Here's how the part is built. I have some questions about the finished solid (model axes, mm). Face numbers are marked on the shaded views. A direction names the side the tool comes from. Round coordinates to 2 decimals unless told otherwise and drop trailing zeros. Write each loop counter-clockwise with the first axis right and the second up, starting at its lowest first coordinate (ties: lowest second). Pieces come first, ordered by that corner, then holes. Notation, with made-up numbers: (37.5, -18) -> (60.5, -18) arc R26 ccw to (60.5, 15) -> close; hole circle Ø2 at (46.5, 3). An arc over 180 degrees is marked (long way). Answer in a Markdown table with one row per item. Add a question column.
from build123d import *

# Parameters (mm, degrees)
F1_DEPTH    = 152.4
F2_T        = 2.54
F2_T3_DEPTH = 157.48


# Not quite as in the source:
# - a shell that OpenCascade refuses in one call is made with other operations: the cavity is built on its own and cut out


with BuildPart() as f1:
    # F0 (on Front) → F1 (new body)
    with BuildSketch(Plane.XZ):
        with BuildLine():
            Line((-37.8300789744, -10.7009902054), (-48.2259040094, -10.7009902054))
            Line((-48.2259040094, -10.7009902054), (-48.2259040094, -7.2357404328))
            ThreePointArc((-48.2259040094, -7.2357404328), (-49.0552526275, -5.8106548767), (-50.7040085729, -5.8277371868))
            Line((-50.7040085729, -5.8277371868), (-59.5905011949, -11.123357617))
            ThreePointArc((-59.5905011949, -11.123357617), (-61.8609001823, -13.4412951055), (-62.6898407936, -16.578236805))
            Line((-62.6898407936, -16.578236805), (-62.6898407936, -27.3817684501))
            Line((-62.6898407936, -27.3817684501), (-43.5946621001, -27.3817684501))
            Line((-43.5946621001, -27.3817684501), (-43.5946621001, -19.9903684501))
            Line((-43.5946621001, -19.9903684501), (0, -19.9903684501))
            Line((0, -19.9903684501), (0, -27.3817684501))
            Line((0, -27.3817684501), (16.9334635139, -27.3817684501))
            Line((16.9334635139, -27.3817684501), (16.9334635139, 48.305941894))
            ThreePointArc((16.9334635139, 48.305941894), (15.0735915744, 52.7960699546), (10.5834635139, 54.655941894))
            Line((10.5834635139, 54.655941894), (6.1501904505, 54.655941894))
            ThreePointArc((6.1501904505, 54.655941894), (2.3177679163, 53.3690474153), (0.0387070827, 50.0299694591))
            Line((0.0387070827, 50.0299694591), (-17.0932790838, -10.7009902054))
            Line((-17.0932790838, -10.7009902054), (-28.2165445387, -10.7009902054))
            Line((-28.2165445387, -10.7009902054), (-28.2165445387, -14.6972788498))
            Line((-28.2165445387, -14.6972788498), (-37.8300789744, -14.6972788498))
            Line((-37.8300789744, -14.6972788498), (-37.8300789744, -10.7009902054))
        make_face()
    extrude(amount=F1_DEPTH)

    # F2: shell of thickness 2.54, made by hand


with BuildPart() as f2_core1:
    # F2_t2: copy of F1
    add(f1.part)

    # the walls: a layer under each face that stays
    f2_faces = [f2_core1.faces().sort_by_distance(p)[0] for p in [
        (-8.5272860005, -76.2, 19.6644896269),
        (-22.6549118113, -76.2, -10.7009902054),
        (-28.2165445387, -76.2, -12.6991345276),
        (-33.0233117566, -76.2, -14.6972788498),
        (-37.8300789744, -76.2, -12.6991345276),
        (-43.0279914919, -76.2, -10.7009902054),
        (-48.2259040094, -76.2, -8.9683653191),
        (-55.1472548839, -76.2, -8.4755474019),
        (-61.8609001823, -76.2, -13.4412951055),
        (-62.6898407936, -76.2, -21.9800026276),
        (-53.1422514468, -76.2, -27.3817684501),
        (-43.5946621001, -76.2, -23.6860684501),
        (-21.79733105, -76.2, -19.9903684501),
        (0, -76.2, -23.6860684501),
        (8.4667317569, -76.2, -27.3817684501),
        (16.9334635139, -76.2, 10.4620867219),
        (15.0735915744, -76.2, 52.7960699546),
        (8.3668269822, -76.2, 54.655941894),
        (2.3177679163, -76.2, 53.3690474153),
    ]]
    thicken(f2_faces, amount=-F2_T, mode=Mode.SUBTRACT)

    # F2_s4 → F2_t3 (cut)
    with BuildSketch(Plane.XZ.offset(-2.54)):
        Polygon((-17.1177250172, -10.6686940951), (-14.6486857366, -11.3906012314), (-15.1706738376, -13.2409902054), (-17.0932790838, -13.2409902054), align=None)
        Polygon((-28.2419445387, -14.6718788498), (-25.6765445387, -14.6972788498), (-25.6765445387, -17.2372788498), (-28.2165445387, -17.2372788498), align=None)
        Polygon((-37.8046789744, -14.6718788498), (-37.8300789744, -17.2372788498), (-40.3700789744, -17.2372788498), (-40.3700789744, -14.6972788498), align=None)
        Polygon((-48.2005040094, -10.6755902054), (-48.2259040094, -13.2409902054), (-50.7659040094, -13.2409902054), (-50.7659040094, -10.7009902054), align=None)
        Polygon((-43.5692621001, -20.0157684501), (-46.1346621001, -19.9903684501), (-46.1346621001, -17.4503684501), (-43.5946621001, -17.4503684501), align=None)
        Polygon((-0.0254, -20.0157684501), (0, -17.4503684501), (2.54, -17.4503684501), (2.54, -19.9903684501), align=None)
    extrude(amount=F2_T3_DEPTH, mode=Mode.SUBTRACT)


with BuildPart() as f1_1:
    add(f1.part)

    # what is left inside the walls is the cavity
    f2_cavity = [f2_core1.part.solids().sort_by_distance(p)[0] for p in [
        (14.368064, -101.6, 11.732087),
    ]]
    add(f2_cavity, mode=Mode.SUBTRACT)


solid = f1_1.part
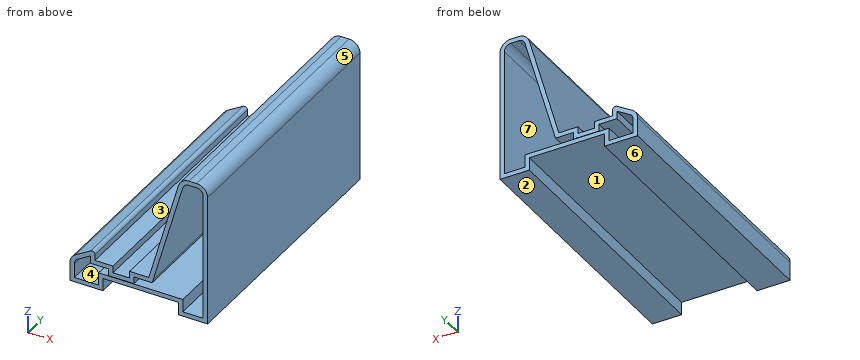
Item 1: On a 3-axis mill with a long thin cutter (end or side, diameter ignored), from which of +Z, -Z, +X, -X, +Y, -Y can I reach the whole of each face in a straight line? I mean the marked faces 1, 2, 3 and 4. Say none if no direction works.
Item 2: I need wall thicknesses on line 1 along X through (y, z) = (-89.5, -23); line 2 along Z through (x, y) = (-22.5, -11); line 3 along X through (y, z) = (-123, -9). Which ranges of each line are inside material? Lowest first, please. Write a range as from..to.
Item 3: If we section it at A-A on x = -2: Please give me the cut outline in (y, z), then the cut area to 3 significant figures.
Item 4: If we mould it in two halves opening along Z, with no side actions, what happens to the marked faces 5, 6 and 7? For each: pulls with the +Z half, pulls with the -Z half, needs draft (parallel to the pull), parting line crosses it, or undercut.
Item 5: For P1, Ø10, axis at x = -15, y = -64.5, coming from the -Z side; P2, Ø3.5, axis at y = -110.5, z = -12, coming from the -X side; P3, Ø11, axis at x = -56, y = -98, coming from the +Z side, each with a flat end and sliding along its axis, tell me the tip position at first contact or that it passes through.
Item 6: If we section it at B-B on z = 2.5: Please give me the cut outline in (x, y).
Results list:
| question | item | result |
|---|---|---|
| 1 | face 1 | -Z, +Y, -Y |
| 1 | face 2 | -Z, +X, -X, +Y, -Y |
| 1 | face 3 | +Z, +Y, -Y |
| 1 | face 4 | +Y, -Y |
| 2 | line 1 | -62.69..-60.15, -46.13..-43.59, 0..2.54, 14.39..16.93 |
| 2 | line 2 | -19.99..-17.45, -13.24..-10.7 |
| 2 | line 3 | -56.03..-51.07, -50.77..-48.23, -16.61..-13.97, 14.39..16.93 |
| 3 | outline | (-152.4, -19.99) -> (0, -19.99) -> (0, -17.45) -> (-152.4, -17.45) -> close; (-152.4, 33.45) -> (0, 33.45) -> (0, 42.8) -> (-152.4, 42.8) -> close |
| 3 | area | 1,810 mm² |
| 4 | face 5 | pulls with the +Z half |
| 4 | face 6 | pulls with the -Z half |
| 4 | face 7 | undercut |
| 5 | P1 | z = -19.99 |
| 5 | P2 | x = -62.03 |
| 5 | P3 | z = -5.72 |
| 6 | outline | (-13.37, -152.4) -> (-10.73, -152.4) -> (-10.73, 0) -> (-13.37, 0) -> close; (14.39, -152.4) -> (16.93, -152.4) -> (16.93, 0) -> (14.39, 0) -> close |
